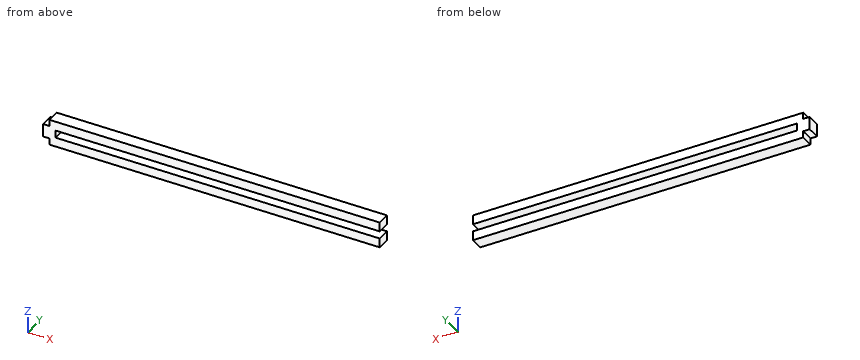
Autodesk Inventor part; units mm, degrees
ref_plane "YZ Plane" through (0, 0, 0) normal (1, 0, 0) x (0, 1, 0)
ref_plane "XZ Plane" through (0, 0, 0) normal (0, 1, 0) x (-1, 0, 0)
ref_plane "XY Plane" through (0, 0, 0) normal (0, 0, 1) x (1, 0, 0)
sketch "Sketch1" plane through (0, 0, 0) normal (0, 1, 0) x (-1, 0, 0)
  line L0 (2.9, 0) -> (2.9, -3)
  line L1 (1.5, 0) -> (2.9, 0)
  line L2 (1.5, 1.4) -> (1.5, 0)
  line L3 (0, 1.4) -> (1.5, 1.4)
  line L4 (0, -4.4) -> (0, 1.4)
  line L5 (1.5, -4.4) -> (0, -4.4)
  line L6 (1.5, -3) -> (1.5, -4.4)
  line L7 (1.5, -3) -> (2.9, -3)
  line L8 (0.1, -4.3) -> (0.1, 1.3)
  line L9 (0.1, 1.3) -> (1.4, 1.3)
  line L10 (1.4, 1.3) -> (1.4, -0.1)
  line L11 (1.4, -0.1) -> (2.8, -0.1)
  line L12 (2.8, -0.1) -> (2.8, -2.9)
  line L13 (2.8, -2.9) -> (1.4, -2.9)
  line L14 (1.4, -2.9) -> (1.4, -4.3)
  line L15 (1.4, -4.3) -> (0.1, -4.3)
  line L16 (0.1, -4.3) -> (-69.9, -4.3)
  line L17 (-69.9, -4.3) -> (-69.9, -2.3)
  line L18 (-69.9, -2.3) -> (0.1, -2.3)
  line L19 (0.1, -2.3) -> (0.1, -4.3)
  line L20 (0.1, 1.3) -> (-69.9, 1.3)
  line L21 (-69.9, 1.3) -> (-69.9, -0.7)
  line L22 (-69.9, -0.7) -> (0.1, -0.7)
  line L23 (0.1, -0.7) -> (0.1, 1.3)
  point P0 (0, 0)
  point P1 (0.1, -0.7)
  point P2 (0.1, -2.3)
  dimension "d0" = 0.1
  dimension "d1" = 1.6
  dimension "d2" = 70
extrude "Extrusion1" add sketch "Sketch1" along normal blind 2.8 contours L20 L8 L22 L4 | L4 L22 L21 L20 | L16 L17 L18 L4 | L4 L18 L8 L16 | L9 L10 L11 L12 L13 L14 L15 L8
equation "\"d0\" = slack"
equation "\"slack\" = 0.1"
equation "\"slack2\" = 0.1"
properties part number "Widełki"
Verification items for the finished model (mm, model axes). Coordinates: 2 decimals unless noted, no trailing zeros. Write each loop counter-clockwise with the first axis right and the second up, starting at its lowest first coordinate (ties: lowest second). Pieces come first, ordered by that corner, then holes. Notation, with made-up numbers: M -39.5,65.25 L -26.5,65.25 A23 ccw -26.5,92.25 Z; hole C 59.5,-2.5 d4. An arc over 180 degrees is marked long. Use CSV: the item, a comma, the result in double quotes.
Q1. Thickness scan on line 1 along Z through (x, y) = (40, 1.5); line 2 along X through (y, z) = (1.35, -2); line 3 along X through (y, z) = (0.7, -4). Record the ranges inside material, lowest first. Write a range as [from, to].
Computed values:
line 1,"[-4.3, -2.3], [-0.7, 1.3]"
line 2,"[-2.8, -0.1]"
line 3,"[-1.4, 69.9]"
Q2. Go/stop test with flat-tipped pins: P1, Ø1.1, axis at y = 1, z = 0.5, coming from the -X side; P2, Ø1.1, axis at x = -2, y = 1.5, coming from the -Z side; P3, Ø1.5, axis at x = 30.5, z = -3.5, coming from the -Y side; P4, Ø1.1, axis at x = -2, y = 1, coming from the +Z side. Record where each tip stops, or that it passes through.
Computed values:
P1,"x = -1.4"
P2,"z = -2.9"
P3,"y = 0"
P4,"z = -0.1"
Q3. Section check B-B, the plane y = 1.6. Enter the section's corners in (x, z), and give its area (3 significant figures).
Computed values:
outline,"M -2.8,-2.9 L -1.4,-2.9 L -1.4,-4.3 L 69.9,-4.3 L 69.9,-2.3 L -0.1,-2.3 L -0.1,-0.7 L 69.9,-0.7 L 69.9,1.3 L -1.4,1.3 L -1.4,-0.1 L -2.8,-0.1 Z"
area,"291 mm²"
Q4. Section check A-A, the plane x = 19. Enter the section's corners in (y, z), and give its area (3 significant figures).
Computed values:
outline,"M 0,-4.3 L 2.8,-4.3 L 2.8,-2.3 L 0,-2.3 Z; M 0,-0.7 L 2.8,-0.7 L 2.8,1.3 L 0,1.3 Z"
area,"11.2 mm²"
Q5. Section check C-C, the plane z = 0.7. Enter the section's corners in (x, y), and give its area (3 significant figures).
Computed values:
outline,"M -1.4,0 L 69.9,0 L 69.9,2.8 L -1.4,2.8 Z"
area,"200 mm²"
